Study the drawing (mm; zero at the part's minimum x, y, z) and answer. A direction names the side the tool comes from. Coordinates: 2 decimals unless noted, no trailing zeros. Order: outer loops, then holes, each group sorted by start corner. A loop starts at its lowest first (then second) coordinate and runs counter-clockwise, first axis right, second up. Notation, with made-up numbers: (25, 37.25) -> (47, 37.25) arc R11 ccw to (47, 51.25) -> close; hole circle Ø4 at (1.5, 46.5). An arc over 180 degrees is marked (long way). Answer in a Markdown table with one row per item. Add a question column.
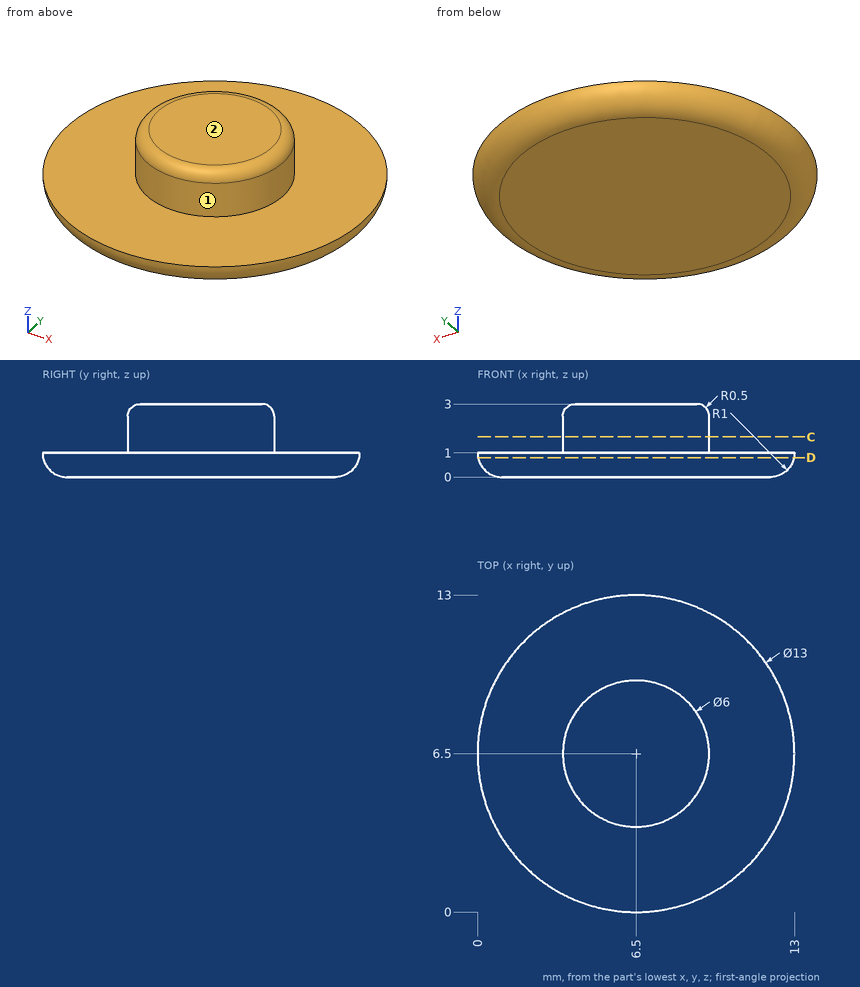
Q1. Straight lines are drawn through the part: line 1 (Z direction, x = 9, y = 9.75); line 2 (Z direction, x = 9.25, y = 1); line 3 (Y direction, x = 9.5, z = 0.65). For each, find the intervals that lie inside material, in ascending order.
Q2. For the marked faces 1 and 2, determine the directions among +Z, -Z, +X, -X, +Y, -Y from which every point of the face is accessible in a straight line to the end or side of a thin tool.
Q3. A cutting plane is placed at C-C (z = 1.65). Determine the outline of the cut face in (x, y), then the cut area to 3 significant figures.
Q4. A cutting plane is placed at D-D (z = 0.8). Determine the outline of the cut face in (x, y).
Returned:
| question | item | result |
|---|---|---|
| 1 | line 1 | z = 0 to 1 |
| 1 | line 2 | z = 0.24 to 1 |
| 1 | line 3 | y = 0.81 to 12.19 |
| 2 | face 1 | +Z |
| 2 | face 2 | +Z, +X, -X, +Y, -Y |
| 3 | outline | circle Ø6 at (6.5, 6.5) |
| 3 | area | 28.3 mm² |
| 4 | outline | circle Ø12.96 at (6.5, 6.5) |
